The model under review builds one solid part; all positions refer to its coordinate system, in mm. A direction names the side the tool comes from. Round coordinates to 2 decimals unless told otherwise and drop trailing zeros. Loops run counter-clockwise (first coordinate to the right, second up) from the corner with the lowest first, then second, coordinate; pieces in that order, holes last. Notation, with made-up numbers: M 5,17 L 44,17 A18 cw 44,31 Z; hole C 78,7 d2. An arc over 180 degrees is marked long. Answer in a Markdown table with one row per item. Add a question column.
from build123d import *

# Parameters (mm, degrees)
SALIENTE_EXTRUIR1_DEPTH = 10
CROQUIS2_R              = 2
CORTAR_EXTRUIR1_DEPTH   = 10


with BuildPart() as part:
    # Croquis1 → Saliente-Extruir1 (new body)
    with BuildSketch(Plane.XY):
        with BuildLine():
            Line((-17.5, 0), (-17.5, -16.507351352))
            Line((-17.5, -16.507351352), (-37.5, -16.507351352))
            Line((-37.5, -16.507351352), (-37.5, -17.007351352))
            Line((-37.5, -17.007351352), (-17, -17.007351352))
            Line((-17, -17.007351352), (-17, 0.5))
            ThreePointArc((-17, 0.5), (0, 17.007351352), (17, 0.5))
            Line((17, 0.5), (17, -17.007351352))
            Line((17, -17.007351352), (37.5, -17.007351352))
            Line((37.5, -17.007351352), (37.5, -16.507351352))
            Line((37.5, -16.507351352), (17.5, -16.507351352))
            Line((17.5, -16.507351352), (17.5, 0))
            ThreePointArc((17.5, 0), (0, 17.5), (-17.5, 0))
        make_face()
    extrude(amount=SALIENTE_EXTRUIR1_DEPTH)

    # Croquis2 → Cortar-Extruir1 (cut)
    with BuildSketch(Plane(origin=(0, -16.507351352, 0), x_dir=(1, 0, 0), z_dir=(0, 1, 0))):
        with Locations(Location((-27.5, -5, 0), (0, 0, 270))):
            Circle(CROQUIS2_R)
        with Locations(Location((27.5, -5, 0), (0, 0, 270))):
            Circle(CROQUIS2_R)
    extrude(amount=-CORTAR_EXTRUIR1_DEPTH, mode=Mode.SUBTRACT)


solid = part.part
1. Mouldability with a two-part tool opening along Z and no side actions: class faces 5 (the cylindrical face through (25.548, -16.754, 4.566)), 6 (the flat face through (-17, -8, 5)) as released by +Z, released by -Z, zero draft, split by the parting line, or undercut.
2. Take a section at C-C, the plane x = -27.5. State the section outline as (y, z) points.
3. For pin 1 Ø1.5 at (y, z) = (-13, 8) entering from -X; pin 2 Ø3 at (y, z) = (-7.5, 4) entering from +X; pin 3 Ø6 at (x, z) = (-7, 4.5) entering from +Y, all flat-tipped, find the tip position at first contact; note any pin that passes through.
4. To check wall thickness, follow probe 1 along X at (y, z) = (-16.9, 5); probe 2 along X at (y, z) = (-12.5, 9.25); probe 3 along Y at (x, z) = (22.5, 5.5). State the ranges of each line that lie inside material, in increasing order.
5. Take a section at D-D, the plane z = 8.5. State the section outline as (x, y) points.
6. Machinability: for faces 1 (the flat face through (17.5, -8, 5)), 2 (the flat face through (-17.5, -8, 5)), 3 (the flat face through (17, -8, 5)), 4 (the cylindrical face through (-29.452, -16.754, 4.566)), which of the approach directions +Z, -Z, +X, -X, +Y, -Y give a long, thin tool a straight path to every point of the face, cutting with its end or side? Answer none if there is none.
7. Take a section at A-A, the plane y = -12. State the section outline as (x, z) points, and give its area (3 significant figures).
Check sheet entries:
| question | item | result |
|---|---|---|
| 1 | face 5 | undercut |
| 1 | face 6 | zero draft |
| 2 | outline | M -17.01,0 L -16.51,0 L -16.51,3 L -17.01,3 Z; M -17.01,7 L -16.51,7 L -16.51,10 L -17.01,10 Z |
| 3 | pin 1 | stops at x = -17.5 |
| 3 | pin 2 | stops at x = 17.5 |
| 3 | pin 3 | stops at y = 17.04 |
| 4 | probe 1 | x = -37.5 to -29.5, -25.5 to -17, 17 to 25.5, 29.5 to 37.5 |
| 4 | probe 2 | x = -17.5 to -17, 17 to 17.5 |
| 4 | probe 3 | y = -17.01 to -16.51 |
| 5 | outline | M -37.5,-17.01 L -17,-17.01 L -17,0.5 A17.01 cw 17,0.5 L 17,-17.01 L 37.5,-17.01 L 37.5,-16.51 L 17.5,-16.51 L 17.5,0 A17.5 ccw -17.5,0 L -17.5,-16.51 L -37.5,-16.51 Z |
| 6 | face 1 | +Z, -Z, +X, +Y |
| 6 | face 2 | +Z, -Z, -X, +Y |
| 6 | face 3 | +Z, -Z, -Y |
| 6 | face 4 | +Y, -Y |
| 7 | outline | M -17.5,0 L -17,0 L -17,10 L -17.5,10 Z; M 17,0 L 17.5,0 L 17.5,10 L 17,10 Z |
| 7 | area | 10.0 mm^2 |
